```python
from build123d import *

# Parameters (mm, degrees)
F1_DEPTH = 139.7
F2_W     = 10.2
F2_H     = 32.6
F3_DEPTH = 150
F4_W     = 6.2
F4_H     = 32.647062
F4_H_2   = 32.911505
F4_H_3   = 34.58407
F4_H_4   = 35.141594
F4_H_5   = 35.977877
F4_H_6   = 40.159295
F5_DEPTH = 150
F6_DEPTH = 150
F7_R     = 2
F7_R_2   = 1.956251
F8_DEPTH = 25


with BuildPart() as f1:
    # F0 (on Front) → F1 (new body)
    with BuildSketch(Plane.XZ):
        Polygon((-24.75, 35.1), (-63.5, 35.1), (-63.5, 0), (63.5, 0), (63.5, 35.1), (24.75, 35.1), (24.75, 5), (-24.75, 5), align=None)
    extrude(amount=F1_DEPTH)

    # F2 (on face) → F3 (cut)
    with BuildSketch(Plane.XZ.offset(139.7)):
        with Locations((-56.4, 18.8)):
            Rectangle(F2_W, F2_H)
        with Locations((56.4, 18.8)):
            Rectangle(F2_W, F2_H)
    extrude(amount=-F3_DEPTH, mode=Mode.SUBTRACT)

    # F4 (on Front) → F5 (cut)
    with BuildSketch(Plane.XZ):
        with Locations((-29.85, 21.323531)):
            Rectangle(F4_W, F4_H)
        with Locations((-38.05, 21.455752)):
            Rectangle(F4_W, F4_H_2)
        with Locations((-46.25, 22.292035)):
            Rectangle(F4_W, F4_H_3)
        with Locations((29.85, 22.570797)):
            Rectangle(F4_W, F4_H_4)
        with Locations((38.05, 22.988938)):
            Rectangle(F4_W, F4_H_5)
        with Locations((46.25, 25.079648)):
            Rectangle(F4_W, F4_H_6)
    extrude(amount=-F5_DEPTH, mode=Mode.SUBTRACT)

    # F4 (on Front) → F6 (cut)
    with BuildSketch(Plane.XZ):
        with Locations((-29.85, 21.323531)):
            Rectangle(F4_W, F4_H)
        with Locations((-38.05, 21.455752)):
            Rectangle(F4_W, F4_H_2)
        with Locations((-46.25, 22.292035)):
            Rectangle(F4_W, F4_H_3)
        with Locations((29.85, 22.570797)):
            Rectangle(F4_W, F4_H_4)
        with Locations((38.05, 22.988938)):
            Rectangle(F4_W, F4_H_5)
        with Locations((46.25, 25.079648)):
            Rectangle(F4_W, F4_H_6)
    extrude(amount=F6_DEPTH, mode=Mode.SUBTRACT)

    # F7 (on face) → F8 (cut)
    with BuildSketch(Plane.XY.offset(2.5)):
        with Locations((-56.4, -6.35)):
            Circle(F7_R)
        with Locations((56.4, -6.35)):
            Circle(F7_R)
        with Locations((-56.4, -69.85)):
            Circle(F7_R_2)
        with Locations((56.4, -69.85)):
            Circle(F7_R)
        with Locations((-56.4, -133.35)):
            Circle(F7_R)
        with Locations((56.4, -133.35)):
            Circle(F7_R)
    extrude(amount=-F8_DEPTH, mode=Mode.SUBTRACT)


solid = f1.part
```
Work out the finished part from the listing and answer in its coordinate system (mm). A direction names the side the tool comes from. Give positions to 0.01 mm unless a question says otherwise; leave off trailing zeros. Loops run counter-clockwise (first coordinate to the right, second up) from the corner with the lowest first, then second, coordinate; pieces in that order, holes last. Notation, with made-up numbers: M 6,86 L 64,86 A23 cw 64,102 Z; hole C -9,54.5 d9. An arc over 180 degrees is marked long. One line per item, written item: value. Start each with the question number.
1. Which of the six approach directions +Z, -Z, +X, -X, +Y, -Y give full straight-line access (tool end or side, diameter ignored) to faces 4 (the face through (-49.35, -69, 20)), 5 (the face through (-63.5, -69, 18))?
2. Find the intervals of material crossed by probe 1 along Y at (x, z) = (-56.4, 1.4); probe 2 along X at (y, z) = (-133, 1); probe 3 along X at (y, z) = (-69, 1), in increasing order.
3. Each of these flat-tipped pins is pushed along its axis until it touches: P1, Ø4, axis at x = -36.5, z = 24, coming from the -Y side; P2, Ø3, axis at x = 54.5, y = -103, coming from the +Z side; P3, Ø1.5, axis at x = 5.5, y = -110.5, coming from the +Z side. Where does it stop, or does it pass through?
4. Find section B-B (x = -13). Give the vertices of the cut face in (y, z), and give its area (4 significant figures).
5. Find section A-A (y = -69.85). State how many separate pieces and enclosed holes the cut face has, and give its area (3 significant figures).
6. Determine the mould class of faces 1 (the face through (63.5, -69, 17)), 2 (the face through (-32.95, -69, 20)), 3 (the face through (-1, -69, 0)) for opening direction X: released by +X, released by -X, zero draft, split by the parting line, or undercut.
Reported:
1. face 4: +Z, +Y, -Y
1. face 5: +Z, -Z, -X, +Y, -Y
2. probe 1: y = -139.7 to -135.35, -131.35 to -71.81, -67.89 to -8.35, -4.35 to 0
2. probe 2: x = -63.5 to -58.37, -54.43 to 54.43, 58.37 to 63.5
2. probe 3: x = -63.5 to -58.16, -54.64 to 54.59, 58.21 to 63.5
3. P1: stops at y = -139.7
3. P2: stops at z = 2.5
3. P3: stops at z = 5
4. outline: M -139.7,0 L 0,0 L 0,5 L -139.7,5 Z
4. area: 698.5 mm²
5. separate pieces: 3
5. enclosed holes: 0
5. area: 1,160 mm²
6. face 1: released by +X
6. face 2: undercut
6. face 3: zero draft
